```python
from build123d import *

# Parameters (mm, degrees)
F1_DEPTH = 82
F2_R     = 5
F3_DEPTH = 48
F5_DEPTH = 14


# Not quite as in the source:
# - a pattern or mirror of a feature is missing from the dataset's text; its kind, count and spacing are read off the source's solid


with BuildPart() as f1:
    # F0 (on Right) → F1 (new body)
    with BuildSketch(Plane.YZ):
        Polygon((12.5, 65), (-12.5, 65), (-20, 29), (-24, 29), (-24, -29), (-20, -29), (-12.5, -75), (12.5, -75), (20, -29), (24, -29), (24, 29), (20, 29), align=None)
    extrude(amount=F1_DEPTH)

    # F2 (on face) → F3 (intersect, through all)
    with BuildSketch(Plane(origin=(0, 24, 0), x_dir=(-1, 0, 0), z_dir=(0, 1, 0))):
        Polygon((-26.5581123827, 75), (-55.4418876173, 75), (-92, 11.6794919243), (-92, -7.5549307949), (-55.8867711433, -85), (-26.1132288567, -85), (10, -7.5549307949), (10, 11.6794919243), align=None)
        with Locations((-41, -57)):
            Circle(F2_R, mode=Mode.SUBTRACT)
        with Locations((-41, 47)):
            Circle(F2_R, mode=Mode.SUBTRACT)
    extrude(amount=-F3_DEPTH, mode=Mode.INTERSECT)

    # F4 (on face) → F5 (cut)
    with BuildSketch(Plane(origin=(0, 24, 0), x_dir=(-1, 0, 0), z_dir=(0, 1, 0))):
        with BuildLine():
            ThreePointArc((-52.3229859469, 45.2858959478), (-48.3869925151, 38.4821097444), (-41, 35.7958683968))
            Line((-41, 35.7958683968), (-41, 66))
            Line((-41, 66), (-56, 66))
            Line((-56, 66), (-52.3229859469, 45.2858959478))
        make_face()
        with BuildLine():
            Line((-41, 66), (-41, 35.7958683968))
            ThreePointArc((-41, 35.7958683968), (-33.6130074849, 38.4821097444), (-29.6770140531, 45.2858959478))
            Line((-29.6770140531, 45.2858959478), (-26, 66))
            Line((-26, 66), (-41, 66))
        make_face()
    f5 = extrude(amount=-F5_DEPTH, mode=Mode.SUBTRACT)

    # F5_copies: F5 across plane
    add(f5.mirror(Plane(origin=(0, 0, 0), x_dir=(0, 0, -1), z_dir=(0, -1, 0))), mode=Mode.SUBTRACT)


solid = f1.part
```
Geometry: final body of the model. Coordinates: model frame, mm. A direction names the side the tool comes from. Coordinates: 2 decimals unless noted, no trailing zeros. Order: outer loops, then holes, each group sorted by start corner. A loop starts at its lowest first (then second) coordinate and runs counter-clockwise, first axis right, second up. Notation, with made-up numbers: (54, 1.5) - (91, 1.5) arc R15 ccw to (91, 25.5) - close; hole circle Ø11 at (-33, 31.25). An arc over 180 degrees is marked (long way). Return JSON: item names as keys, results as strings. Group by question number.
1. Cut plane C-C (x = 7). Output: boundary loops of the cut face in (y, z), plus the area to 3 significant figures.
2. Pull-direction query (Y, two-part tool) for faces 6 (the face through (40.426, -17.136, -46.567)), 7 (the face through (0, 0, 0)), 8 (the face through (40, 24, 0)); classes: pulls with the +Y half, pulls with the -Y half, needs draft (parallel to the pull), parting line crosses it, or undercut.
3. Set-up query: faces 1 (the face through (41, 10, 54)), 2 (the face through (40, -22, -29)), 3 (the face through (41, -10, 54)), 4 (the face through (40, 22, 29)), 5 (the face through (40, 22, -29)). Return all of +Z, -Z, +X, -X, +Y, -Y with unobstructed straight access to the full face (end or side cutting, diameter ignored); none if empty.
4. Cut plane A-A (y = 7). Output: boundary loops of the cut face in (x, z), plus the area to 3 significant figures.
5. Pin query (flat end, axial travel): pin 1 (2 mm diameter, centred on x = 52, y = -22, fed in from +Z); pin 2 (9 mm diameter, centred on x = 37, z = 48, fed in from +Y); pin 3 (1.2 mm diameter, centred on x = 48, y = 21, fed in from -Z). Return the tip coordinate at first contact, or that it passes through.
6. Material intervals for line 1 along Z through (x, y) = (41, -3.5); line 2 along X through (y, z) = (-4, -37); line 3 along X through (y, z) = (6.5, -43), sorted ascending. Write a range as [from, to].
7. Cut plane D-D (z = 47). Output: boundary loops of the cut face in (x, y), plus the area to 3 significant figures.
8. Cut plane B-B (z = -57). Output: boundary loops of the cut face in (x, y), plus the area to 3 significant figures.
Resolved:
{
 "1": {"outline": "(-24, -29) - (-20, -29) - (-17.55, -44.01) - (17.55, -44.01) - (20, -29) - (24, -29) - (24, 29) - (20, 29) - (17.47, 41.12) - (-17.47, 41.12) - (-20, 29) - (-24, 29) - close", "area": "3,800 mm²"},
 "2": {"face 6": "pulls with the -Y half", "face 7": "needs draft", "face 8": "pulls with the +Y half"},
 "3": {"face 1": "+Z, +Y", "face 2": "-Z, +X, -X, -Y", "face 3": "+Z, -Y", "face 4": "+Z, +X, -X, +Y", "face 5": "-Z, +X, -X, +Y"},
 "4": {"outline": "(0, -29) - (21.45, -75) - (60.55, -75) - (82, -29) - (82, 29) - (61.22, 65) - (20.78, 65) - (0, 29) - close; hole circle Ø10 at (41, -57); hole circle Ø10 at (41, 47)", "area": "9,590 mm²"},
 "5": {"pin 1": "stops at z = 29", "pin 2": "stops at y = 10", "pin 3": "stops at z = -29"},
 "6": {"line 1": "z = [-75, -62], [-52, 42], [52, 65]", "line 2": "x = [3.73, 78.27]", "line 3": "x = [6.53, 75.47]"},
 "7": {"outline": "(10.39, -16.25) - (29.37, -16.25) - (29.37, -10) - (36, -10) - (36, 10) - (29.37, 10) - (29.37, 16.25) - (10.39, 16.25) - close; (46, -10) - (52.63, -10) - (52.63, -16.25) - (71.61, -16.25) - (71.61, 16.25) - (52.63, 16.25) - (52.63, 10) - (46, 10) - close", "area": "1,500 mm²"},
 "8": {"outline": "(13.06, -15.43) - (36, -15.43) - (36, 15.43) - (13.06, 15.43) - close; (46, -15.43) - (68.94, -15.43) - (68.94, 15.43) - (46, 15.43) - close", "area": "1,420 mm²"}
}
